Answer from the drawing. Dimensions are ordinates in mm from the lowest x, y and z of the part. A direction names the side the tool comes from. Give positions to 0.01 mm unless a question says otherwise; leave off trailing zeros. Write each loop counter-clockwise with the first axis right and the second up, starting at its lowest first coordinate (ties: lowest second). Pieces come first, ordered by that corner, then holes. Notation, with made-up numbers: (-32.75, -9.75) -> (-2.75, -9.75) arc R14 ccw to (-2.75, 10.25) -> close; hole circle Ø10 at (8.5, 84.25). An arc over 180 degrees is marked (long way). Put each result on its own line as item: value. Start each with the question number.
1) A cutting plane is placed at C-C (y = 16). Write down the section's boundary in (x, z).
2) A cutting plane is placed at D-D (x = 48). Write down the section's boundary in (y, z), then the cut area to 3 significant figures.
3) A cutting plane is placed at A-A (y = 35). Write down the section's boundary in (x, z), then the cut area to 3 significant figures.
4) For the marked faces 4, 5 and 6, determine the directions among +Z, -Z, +X, -X, +Y, -Y from which every point of the face is accessible in a straight line to the end or side of a thin tool.
5) For a pull along X with two mould halves and no side action, classify the marked faces 1, 2 and 3 as released by +X, released by -X, zero draft, split by the parting line, or undercut.
6) Flat-ended cylindrical pins translate along their axes: pin 1 Ø1 at (x, z) = (100, 4) entering from -Y; pin 2 Ø4 at (y, z) = (67, 5) entering from +X; pin 3 Ø8 at (y, z) = (30, 8) entering from -X; pin 4 Ø12 at (x, z) = (134, 15) entering from +Y. Find the tip coordinate at first contact, or state that the pin passes through.
7) Find the intervals of material crossed by line 1 along Z through (x, y) = (73.5, 75); line 2 along X through (y, z) = (25.5, 6.5) (1 decimal); line 3 along X through (y, z) = (5.5, 6), in increasing order. Write a range as from..to.
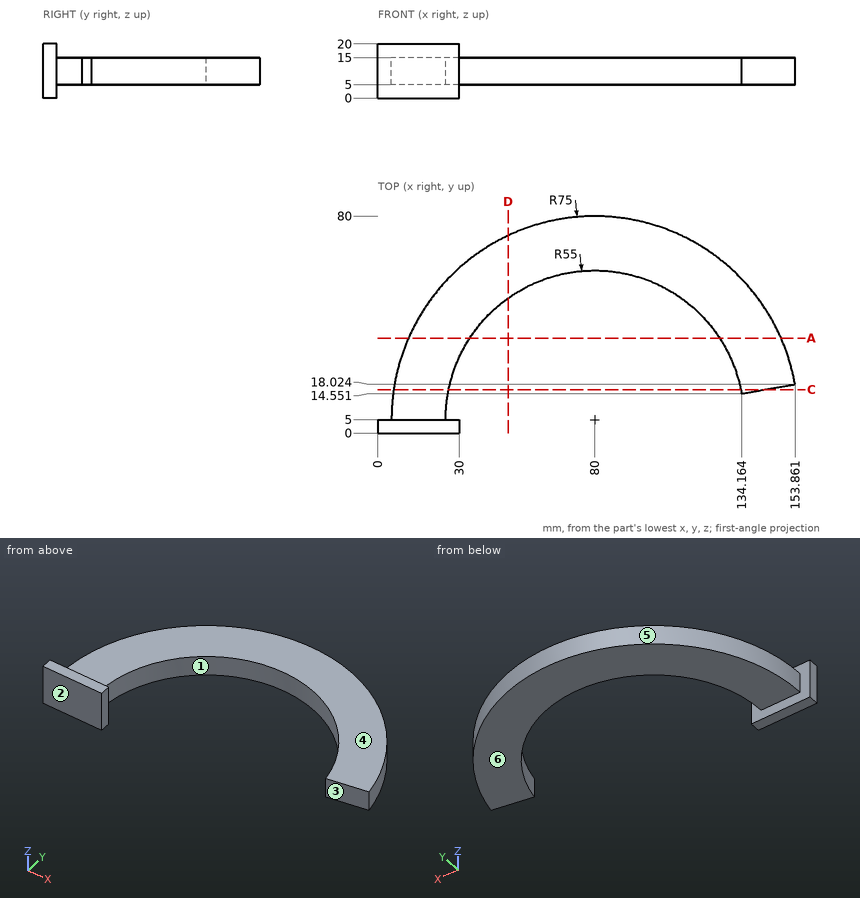
Reply:
1. outline: (5.81, 5) -> (26.11, 5) -> (26.11, 15) -> (5.81, 15) -> close; (133.89, 5) -> (142.38, 5) -> (142.38, 15) -> (133.89, 15) -> close
2. outline: (49.73, 5) -> (72.83, 5) -> (72.83, 15) -> (49.73, 15) -> close
2. area: 231 mm2
3. outline: (11.26, 5) -> (33.9, 5) -> (33.9, 15) -> (11.26, 15) -> close; (126.1, 5) -> (148.74, 5) -> (148.74, 15) -> (126.1, 15) -> close
3. area: 453 mm2
4. face 4: +Z, +X, -X, +Y
4. face 5: +Z, -Z, +Y
4. face 6: -Z, +X, -X, +Y
5. face 1: undercut
5. face 2: zero draft
5. face 3: released by +X
6. pin 1: passes through
6. pin 2: stops at x = 125
6. pin 3: stops at x = 8
6. pin 4: stops at y = 62.63
7. line 1: z = 5..15
7. line 2: x = 7.9..29, 131..152.1
7. line 3: x = 5..25
